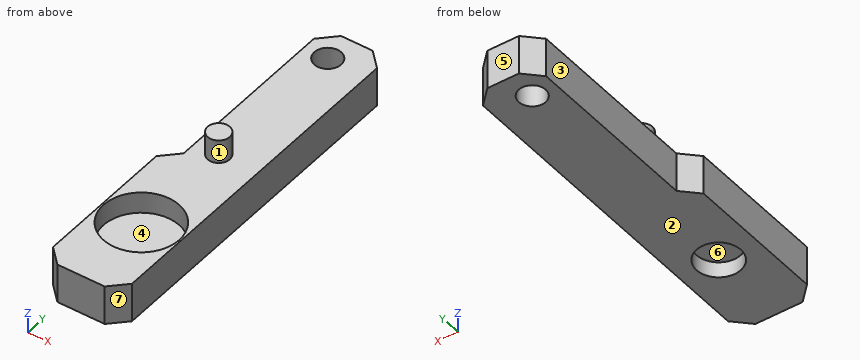
```python
from build123d import *

# Parameters (mm, degrees)
F0_W     = 8
F0_H     = 26.7
F0_R     = 1.4
F0_R_2   = 1.7
F0_R_3   = 4.8
F1_DEPTH = 5
F2_DEPTH = 8
F0_R_4   = 2.8
F3_DEPTH = 2.3
F4_START = 2
F4_DEPTH = 0.3
F5_SIZE  = 1.99999


# Not quite as in the source:
# - a fillet or chamfer is up to 0.001 mm smaller than in the source, because OpenCascade refuses the exact size


with BuildPart() as f1:
    # F0 (on Top) → F1 (new body)
    with BuildSketch(Plane.XY):
        with Locations((1, 4.0926239572)):
            Rectangle(F0_W, F0_H)
        with Locations((0, -5.2573760428)):
            Circle(F0_R, mode=Mode.SUBTRACT)
        with Locations((0, 13.7426239572)):
            Circle(F0_R_2, mode=Mode.SUBTRACT)
        Polygon((-5, -9.2573760428), (-5, -29.2573760428), (5, -29.2573760428), (5, -9.2573760428), (-3, -9.2573760428), align=None)
        with Locations((0, -18.7472271925)):
            Circle(F0_R_3, mode=Mode.SUBTRACT)
    extrude(amount=F1_DEPTH)

    # F0 (on Top) → F2 (join)
    with BuildSketch(Plane.XY):
        with Locations((0, -5.2573760428)):
            Circle(F0_R)
    extrude(amount=F2_DEPTH)

    # F0 (on Top) → F3 (join)
    with BuildSketch(Plane.XY):
        with Locations((0, -18.7472271925)):
            Circle(F0_R_3)
        with Locations((0, -18.7472271925)):
            Circle(F0_R_4, mode=Mode.SUBTRACT)
    extrude(amount=F3_DEPTH)

    # F0 (on Top) → F4 (join)
    with BuildSketch(Plane.XY.offset(F4_START)):
        with Locations((0, -18.7472271925)):
            Circle(F0_R_4)
    extrude(amount=F4_DEPTH)

    # F5 (size 2 in the source; OpenCascade refuses exactly that, so slightly less here)
    f5_edges = [f1.edges().sort_by_distance(p)[0] for p in [
        (-3, -9.257376, 2.5),
        (-3, 17.442624, 2.5),
        (5, 17.442624, 2.5),
        (5, -29.257376, 2.5),
        (-5, -29.257376, 2.5),
    ]]
    chamfer(f5_edges, length=F5_SIZE)


solid = f1.part
```
Verification items for the finished model (mm, model axes). Face numbers are marked on the shaded views. A direction names the side the tool comes from. Coordinates: 2 decimals unless noted, no trailing zeros. Write each loop counter-clockwise with the first axis right and the second up, starting at its lowest first coordinate (ties: lowest second). Pieces come first, ordered by that corner, then holes. Notation, with made-up numbers: M 29,-36 L 71,-36 A20 ccw 71,-5 Z; hole C -33.75,-25.5 d4. An arc over 180 degrees is marked long. Answer as a JSON object with one key per item and string values. Group by question number.
(1) Release check for a two-part mould opening along X. For the marked faces 4, 5, 6 and 7 record: +X half, -X half, draft (parallel to the pull), parting line (faces both ways), or undercut.
(2) Tool access check on the marked faces 1, 2 and 3. Record the directions out of +Z, -Z, +X, -X, +Y, -Y that give a thin tool (end or side, any length) a straight path to the whole face; none if there is none.
(3) Cross-section at A-A, the plane x = 0. Record the cut outline in (y, z), and give its area (3 significant figures).
(4) Gauge pin test, flat ends, axial feed: pin 1 (5 mm diameter, centred on x = -1.5, y = 5.5, fed in from +Z); pin 2 (5 mm diameter, centred on x = 0.5, y = -20.5, fed in from +Z); pin 3 (2.5 mm diameter, centred on y = 4, z = 3, fed in from -X); pin 4 (3 mm diameter, centred on x = 0, y = 13.74, fed in from -Z). Record the tip position at first contact, or that the pin passes through.
(5) Cross-section at B-B, the plane y = -26. Record the cut outline in (x, z), and give its area (3 significant figures).
(6) Material ranges on line 1 (Y direction, x = 0, z = 4.35); line 2 (Y direction, x = 0, z = 1.1); line 3 (Z direction, x = 2.25, y = -16.5), recorded low to high.
(7) Cross-section at C-C, the plane x = 4. Record the cut outline in (y, z).
(8) Cross-section at D-D, the plane z = 6. Record the cut outline in (x, y), and give its area (3 significant figures).
Reply:
{
 "1": {"face 4": "undercut", "face 5": "draft", "face 6": "undercut", "face 7": "+X half"},
 "2": {"face 1": "+Z", "face 2": "-Z, +X, -X, +Y, -Y", "face 3": "+Z, -Z, -X, +Y"},
 "3": {"outline": "M -29.26,0 L -21.55,0 L -21.55,2 L -15.95,2 L -15.95,0 L 12.04,0 L 12.04,5 L -3.86,5 L -3.86,8 L -6.66,8 L -6.66,5 L -13.95,5 L -13.95,2.3 L -23.55,2.3 L -23.55,5 L -29.26,5 Z; M 15.44,0 L 17.44,0 L 17.44,5 L 15.44,5 Z", "area": "188 mm²"},
 "4": {"pin 1": "z = 5", "pin 2": "z = 2.3", "pin 3": "x = -3", "pin 4": "through"},
 "5": {"outline": "M -5,0 L 5,0 L 5,5 L -5,5 Z", "area": "50.0 mm²"},
 "6": {"line 1": "-29.26 to -23.55, -13.95 to 12.04, 15.44 to 17.44", "line 2": "-29.26 to -21.55, -15.95 to 12.04, 15.44 to 17.44", "line 3": "0 to 2.3"},
 "7": {"outline": "M -28.26,0 L 16.44,0 L 16.44,5 L -16.09,5 L -16.09,2.3 L -21.4,2.3 L -21.4,5 L -28.26,5 Z"},
 "8": {"outline": "C 0,-5.26 d2.8", "area": "6.16 mm²"}
}
